Check sheet for the modelled part. Datum: model origin and axes. Units: mm. Face numbers are marked on the shaded views. Give positions to 0.01 mm unless a question says otherwise; leave off trailing zeros. Loops run counter-clockwise (first coordinate to the right, second up) from the corner with the lowest first, then second, coordinate; pieces in that order, holes last. Notation, with made-up numbers: (9, 17) - (38, 17) arc R37 ccw to (38, 54) - close; hole circle Ø3 at (17.5, -37). An arc over 180 degrees is marked (long way). Use one line per item in the form item = value.
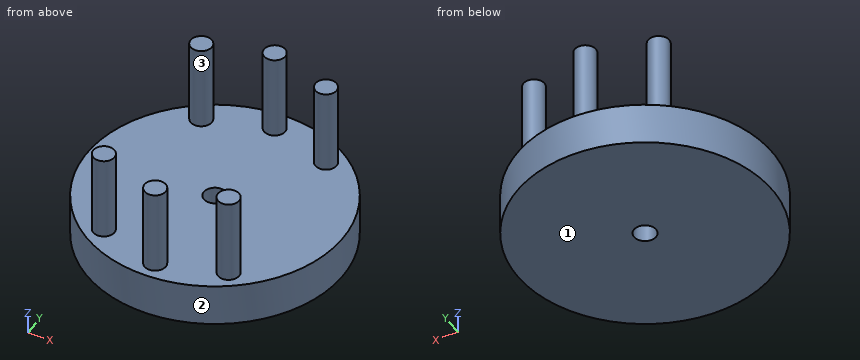
from build123d import *

# Parameters (mm, degrees)
F0_R     = 38.1
F1_DEPTH = 12.7
F2_R     = 3.175
F3_DEPTH = 25.4
F4_R     = 3.175
F5_DEPTH = 25.4
F6_R     = 3.302
F7_DEPTH = 12.7


with BuildPart() as f1:
    # F0 (on Top) → F1 (new body)
    with BuildSketch(Plane.XY):
        Circle(F0_R)
    extrude(amount=F1_DEPTH)

    # F2 (on face) → F3 (join)
    with BuildSketch(Plane.XY.offset(12.7)):
        with Locations((0, 32.385)):
            Circle(F2_R)
        with Locations((-18.753842, 26.402304)):
            Circle(F2_R)
        with Locations((18.753842, 26.402304)):
            Circle(F2_R)
    extrude(amount=F3_DEPTH)

    # F4 (on face) → F5 (join)
    with BuildSketch(Plane.XY.offset(12.7)):
        with Locations((-18.753842, -26.402304)):
            Circle(F4_R)
        with Locations((0, -32.385)):
            Circle(F4_R)
        with Locations((18.753842, -26.402304)):
            Circle(F4_R)
    extrude(amount=F5_DEPTH)

    # F6 (on face) → F7 (cut)
    with BuildSketch(Plane.XY.offset(12.7)):
        Circle(F6_R)
    extrude(amount=-F7_DEPTH, mode=Mode.SUBTRACT)


solid = f1.part
Item 1: Section check B-B on x = 0. Record the boundary of the cut face in (y, z).
Answer block:
outline = (-38.1, 0) - (-3.3, 0) - (-3.3, 12.7) - (-29.21, 12.7) - (-29.21, 38.1) - (-35.56, 38.1) - (-35.56, 12.7) - (-38.1, 12.7) - close; (3.3, 0) - (38.1, 0) - (38.1, 12.7) - (35.56, 12.7) - (35.56, 38.1) - (29.21, 38.1) - (29.21, 12.7) - (3.3, 12.7) - close
Item 2: Section check A-A on y = 0. Record the boundary of the cut face in (x, z), then the cut area to 3 significant figures.
Answer block:
outline = (-38.1, 0) - (-3.3, 0) - (-3.3, 12.7) - (-38.1, 12.7) - close; (3.3, 0) - (38.1, 0) - (38.1, 12.7) - (3.3, 12.7) - close
area = 884 mm2
Item 3: Mould release check, pull along Y, two halves, no side actions. Record for the marked faces 1, 2 and 3: released by +Y, released by -Y, zero draft, split by the parting line, or undercut.
Answer block:
face_1 = zero draft
face_2 = split by the parting line
face_3 = undercut
Item 4: Thickness scan on L1, parallel to Y at x = 0, z = 8; L2, parallel to Z at x = -26.5, y = -20.5; L3, parallel to Y at x = 1, z = 6. Record the ranges inside material, lowest first.
Answer block:
L1 = -38.1 to -3.3, 3.3 to 38.1
L2 = 0 to 12.7
L3 = -38.09 to -3.15, 3.15 to 38.09
Item 5: Gauge pin test, flat ends, axial feed: P1, Ø3, axis at x = 19.5, z = 20.5, coming from the +Y side; P2, Ø23, axis at x = -2.5, y = -12, coming from the +Z side; P3, Ø3, axis at y = 29, z = 9.5, coming from the -X side. Record the tip position at first contact, or that the pin passes through.
Answer block:
P1 = 29.58
P2 = 12.7
P3 = -26.37
Item 6: Section check D-D on y = -28. Record the boundary of the cut face in (x, z), then the cut area to 3 significant figures.
Answer block:
outline = (-25.84, 0) - (25.84, 0) - (25.84, 12.7) - (21.5, 12.7) - (21.5, 38.1) - (16.01, 38.1) - (16.01, 12.7) - (-16.01, 12.7) - (-16.01, 38.1) - (-21.5, 38.1) - (-21.5, 12.7) - (-25.84, 12.7) - close
area = 935 mm2
Item 7: Section check C-C on z = 3. Record the boundary of the cut face in (x, y), then the cut area to 3 significant figures.
Answer block:
outline = circle Ø76.2 at (0, 0); hole circle Ø6.6 at (0, 0)
area = 4,530 mm2
